Check sheet for the modelled part. Datum: model origin and axes. Units: mm. A direction names the side the tool comes from. Round coordinates to 2 decimals unless told otherwise and drop trailing zeros. Loops run counter-clockwise (first coordinate to the right, second up) from the corner with the lowest first, then second, coordinate; pieces in that order, holes last. Notation, with made-up numbers: (35.5, 74.5) -> (63.5, 74.5) arc R22 ccw to (63.5, 99.5) -> close; hole circle Ø4 at (89.5, -11). An arc over 180 degrees is marked (long way). Use one line per item in the form item = value. Start each with the question number.
(1) Sectioned sample at B-B (z = 0). Record the cut outline in (x, y), and give its area (3 significant figures).
(2) Draft check along X on faces 5 (the flat face through (6, -3, 38.1)), 6 (the flat face through (-51.968, -3, -19)), 7 (the flat face through (-25.4, -3, -31)), 8 (the flat face through (-51.968, -3, 19)). Enter one of: released by +X, released by -X, zero draft, split by the parting line, or undercut.
(3) Set-up check for faces 1 (the flat face through (-48, -3, 10.16)), 2 (the flat face through (-45, -3, -20.447)), 3 (the flat face through (-46.203, -3, 22)), 4 (the flat face through (-36, -3, 22.86)): record each of +Z, -Z, +X, -X, +Y, -Y from which the full face is reachable in a straight line by a thin tool's end or side.
(4) Sectioned sample at A-A (x = 0). Record the cut outline in (y, z).
(5) Go/stop test with flat-tipped pins: pin 1 (1.9 mm diameter, centred on x = -39.5, y = -2.5, fed in from +Z); pin 2 (1.9 mm diameter, centred on x = -52, y = -2.5, fed in from -Z); pin 3 (3 mm diameter, centred on y = -2, z = 3, fed in from -X). Record where each tip stops, or that it passes through.
(6) Material ranges on probe 1 along X at (y, z) = (-4.5, 0); probe 2 along Z at (x, y) = (-49, -3.25), recorded low to high. Write a range as [from, to].
from build123d import *

# Parameters (mm, degrees)
SKETCH1_R           = 20.32
BOSS_EXTRUDE1_DEPTH = 6.35


with BuildPart() as part:
    # Sketch1 → Boss-Extrude1 (new body)
    with BuildSketch(Plane(origin=(0, 0, 0), x_dir=(1, 0, 0), z_dir=(0, 1, 0))):
        Polygon((-25.4, -38.1), (38.1, -38.1), (38.1, 38.1), (-25.4, 38.1), (-25.4, 22.86), (-38.1, 22.86), (-46.2026, 22.86), (-46.2026, 20.447), (-44.0944, 20.447), (-44.0944, 17.78), (-51.9684, 17.78), (-51.9684, 20.447), (-49.8602, 20.447), (-49.8602, 22.86), (-57.9628, 22.86), (-57.9628, 10.16), (-38.1, 10.16), (-38.1, -10.16), (-57.9628, -10.16), (-57.9628, -22.86), (-49.8602, -22.86), (-49.8602, -20.447), (-51.9684, -20.447), (-51.9684, -17.78), (-44.0944, -17.78), (-44.0944, -20.447), (-46.2026, -20.447), (-46.2026, -22.86), (-38.1, -22.86), (-25.4, -22.86), align=None)
        Circle(SKETCH1_R, mode=Mode.SUBTRACT)
    extrude(amount=-BOSS_EXTRUDE1_DEPTH)


solid = part.part
Checks:
q1.outline = (-38.1, -6.35) -> (-20.32, -6.35) -> (-20.32, 0) -> (-38.1, 0) -> close; (20.32, -6.35) -> (38.1, -6.35) -> (38.1, 0) -> (20.32, 0) -> close
q1.area = 226 mm2
q2.face_5 = zero draft
q2.face_6 = undercut
q2.face_7 = released by -X
q2.face_8 = undercut
q3.face_1 = -X, +Y, -Y
q3.face_2 = +Y, -Y
q3.face_3 = +Z, +Y, -Y
q3.face_4 = +Z, -X, +Y, -Y
q4.outline = (-6.35, -38.1) -> (0, -38.1) -> (0, -20.32) -> (-6.35, -20.32) -> close; (-6.35, 20.32) -> (0, 20.32) -> (0, 38.1) -> (-6.35, 38.1) -> close
q5.pin_1 = 22.86
q5.pin_2 = -22.86
q5.pin_3 = -38.1
q6.probe_1 = [-38.1, -20.32], [20.32, 38.1]
q6.probe_2 = [-17.78, -10.16], [10.16, 17.78]
